Check sheet for the modelled part. Datum: model origin and axes. Units: mm. A direction names the side the tool comes from. Give positions to 0.01 mm unless a question says otherwise; leave off trailing zeros. Loops run counter-clockwise (first coordinate to the right, second up) from the corner with the lowest first, then second, coordinate; pieces in that order, holes last. Notation, with made-up numbers: (75, 30) - (97, 30) arc R37 ccw to (97, 68) - close; hole circle Ø3 at (81.5, 70). An arc over 180 degrees is marked (long way). Use CSV: the item, a comma, the result in double quotes.
Autodesk Inventor part; units mm, degrees
ref_plane "YZ Plane" through (0, 0, 0) normal (1, 0, 0) x (0, 1, 0)
ref_plane "XZ Plane" through (0, 0, 0) normal (0, 1, 0) x (-1, 0, 0)
ref_plane "XY Plane" through (0, 0, 0) normal (0, 0, 1) x (1, 0, 0)
sketch "スケッチ1" plane through (0, 0, 0) normal (0, 0, 1) x (1, 0, 0)
  circle A0 centre (0, 0) radius 21.2
  dimension "d0" = 42.4
extrude "押し出し1" add sketch "スケッチ1" against normal blind 5
sketch "スケッチ2" plane through (0, 0, -5) normal (0, 0, -1) x (-1, 0, 0)
  circle A0 centre (0, 0) radius 22.5
  dimension "d3" = 45
extrude "押し出し2" add sketch "スケッチ2" along normal blind 30
sketch "スケッチ3" plane through (0, 0, -35) normal (0, 0, -1) x (-1, 0, 0)
  circle A0 centre (0, 0) radius 21.2
  dimension "d6" = 42.4
extrude "押し出し3" add sketch "スケッチ3" along normal blind 28
fillet "フィレット1" radius 3 1 edges at (-21.2, 0, 0)
sketch "スケッチ4" plane through (0, 0, -63) normal (0, 0, -1) x (-1, 0, 0)
  line L0 (-1.75, 18.5) -> (1.75, 18.5)
  line L1 (1.75, 18.5) -> (1.75, 17.5)
  line L2 (1.75, 17.5) -> (-1.75, 17.5)
  line L3 (-1.75, 17.5) -> (-1.75, 18.5)
  line L4 (-1.75, -17.5) -> (1.75, -17.5)
  line L5 (1.75, -17.5) -> (1.75, -18.5)
  line L6 (1.75, -18.5) -> (-1.75, -18.5)
  line L7 (-1.75, -18.5) -> (-1.75, -17.5)
  point P0 (0, 0)
  dimension "d10" = 3.5
  dimension "d11" = 1
  dimension "d12" = 3.5
  dimension "d13" = 1
  dimension "d14" = 17.5
  dimension "d15" = 17.5
  dimension "d16" = 1.75
extrude "押し出し4" add sketch "スケッチ4" along normal blind 9
sketch "スケッチ5" plane through (0, 0, 0) normal (0, 0, 1) x (1, 0, 0)
  circle A0 centre (0, 0) radius 21
  dimension "d19" = 42
extrude "押し出し5" add sketch "スケッチ5" along normal blind 45.9
chamfer "面取り1" distance 0.5 angle 45 1 edges at (-21, 0, 45.9)
sketch "スケッチ6" plane through (0, 0, 45.9) normal (0, 0, 1) x (1, 0, 0)
  arc A0 (4.6676, 11.5958) -> (-11.5958, -4.6676) centre (0, 0) ccw
  line L0 (4.6676, 11.5958) -> (11.5958, 4.6676)
  line L1 (-11.5958, -4.6676) -> (-4.6676, -11.5958)
  line L2 (11.5958, 4.6676) -> (9.2337, 4.6676) construction
  arc A1 (11.5958, 4.6676) -> (4.6676, 11.5958) centre (0, 0) ccw construction
  arc A2 (-11.5958, -4.6676) -> (-4.6676, -11.5958) centre (0, 0) ccw construction
  arc A3 (-4.6676, -11.5958) -> (11.5958, 4.6676) centre (0, 0) ccw
  dimension "d25" = 25
  dimension "d26" = 11.5
  dimension "d27" = 23
  dimension "d28" = 45
extrude "押し出し6" add sketch "スケッチ6" along normal blind 2
sketch "スケッチ7" plane through (0, 0, 47.9) normal (0, 0, 1) x (1, 0, 0)
  circle A0 centre (0, 0) radius 4
  dimension "d31" = 8
extrude "押し出し7" add sketch "スケッチ7" along normal blind 20
sketch "スケッチ8" plane through (0, 0, 67.9) normal (0, 0, 1) x (1, 0, 0)
  circle A0 centre (0, 0) radius 4
  arc A1 (-2.6458, 3) -> (2.6458, 3) centre (0, 0) ccw
  line L0 (-2.6458, 3) -> (2.6458, 3)
  point P0 (2.6458, 3)
  dimension "d34" = 3
extrude "押し出し8" cut sketch "スケッチ8" against normal blind 12 contours L0 A0 picked at (-0.6179, 3.1815)
sketch "スケッチ9" plane through (0, 0, 45.9) normal (0, 0, 1) x (1, 0, 0)
  circle A0 centre (0, 17.5) radius 1.75
  circle A1 centre (-17.5, 0) radius 1.75
  circle A2 centre (0, -17.5) radius 1.75
  circle A3 centre (17.5, 0) radius 1.75
  point P0 (0, 0)
  dimension "d37" = 3.5
  dimension "d38" = 17.5
  dimension "d41" = 360
extrude "押し出し9" cut sketch "スケッチ9" against normal blind 12
properties part number "RS-775GM104 v1"
1. Sectioned sample at A-A, the plane z = -61. Record the boundary of the cut face in (x, y), and give its area (3 significant figures).
Completed:
outline,"circle Ø42.4 at (0, 0)"
area,"1,410 mm²"
2. Set-up check for faces 4 (the face through (-8.18, -8.083, 46.886)), 5 (the face through (0, 18.5, -67)), 6 (the face through (-0.228, -15.765, 39.984)), 7 (the face through (-3, 19, 0)), 8 (the face through (0, 17.5, -67)): record each of +Z, -Z, +X, -X, +Y, -Y from which the full face is reachable in a straight line by a thin tool's end or side.
Completed:
face 4,"+Z, -X, -Y"
face 5,"-Z, +X, -X, +Y"
face 6,"+Z"
face 7,"none"
face 8,"-Z, +X, -X"
3. Sectioned sample at B-B, the plane z = 2. Record the boundary of the cut face in (x, y), and give its area (3 significant figures).
Completed:
outline,"circle Ø42 at (0, 0)"
area,"1,390 mm²"
4. Scan lines: line 1 along Y through (x, z) = (0, 36.75); line 2 along Y through (x, z) = (17.5, 43.25); line 3 along X through (y, z) = (-0.5, -35.5). Record each from-to range of solid material in increasing order.
Completed:
line 1,"y = -21 to -19.25, -15.75 to 15.75, 19.25 to 21"
line 2,"y = -11.61 to -1.75, 1.75 to 11.61"
line 3,"x = -21.19 to 21.19"
5. Release check for a two-part mould opening along X. For faces 1 (the face through (-8.982, 8.693, 46.886)), 2 (the face through (8.083, 8.18, 46.886)), 3 (the face through (0, 18, 33.9)) record: released by +X, released by -X, zero draft, split by the parting line, or undercut.
Completed:
face 1,"split by the parting line"
face 2,"released by +X"
face 3,"undercut"
6. Go/stop test with flat-tipped pins: pin 1 Ø3 at (x, z) = (-7.5, -11.5) entering from -Y; pin 2 Ø1.5 at (x, y) = (-17, 15) entering from +Z; pin 3 Ø1 at (x, y) = (-14.5, 14.5) entering from +Z. Record where each tip stops, or that it passes through.
Completed:
pin 1,"stops at y = -21.69"
pin 2,"stops at z = -5"
pin 3,"stops at z = 45.9"
